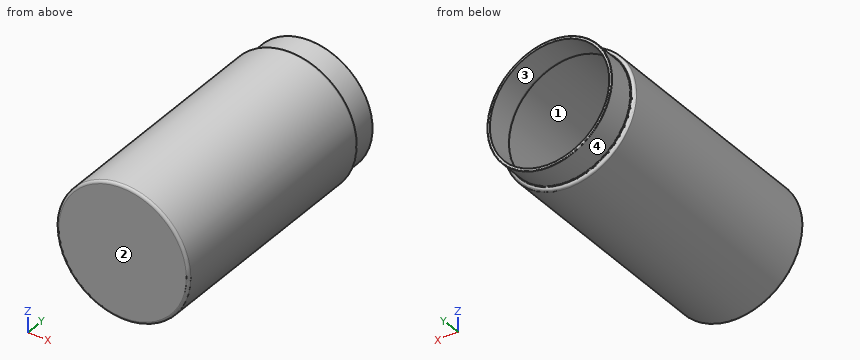
from build123d import *

# Parameters (mm, degrees)
SKETCH1_R           = 25
BOSS_EXTRUDE1_DEPTH = 90
SKETCH2_R           = 23.5
BOSS_EXTRUDE2_DEPTH = 10
FILLET1_R           = 1
FILLET2_R           = 0.2


# Read off the part's stored shape, not the designer's step: Shell1
with BuildPart() as part:
    # Sketch1 → Boss-Extrude1 (new body)
    with BuildSketch(Plane(origin=(0, 0, 0), x_dir=(1, 0, 0), z_dir=(0, 1, 0))):
        with Locations(Location((0, 0, 0), (0, 0, 90))):
            Circle(SKETCH1_R)
    extrude(amount=BOSS_EXTRUDE1_DEPTH)

    # Sketch2 → Boss-Extrude2 (add)
    with BuildSketch(Plane(origin=(0, 90, 0), x_dir=(1, 0, 0), z_dir=(0, 1, 0))):
        with Locations(Location((0, 0, 0), (0, 0, 270))):
            Circle(SKETCH2_R)
    extrude(amount=BOSS_EXTRUDE2_DEPTH)

    # Fillet1
    fillet1_edges = [part.edges().sort_by_distance(p)[0] for p in [
        (0, 0, 25),
        (0, 90, 25),
    ]]
    fillet(fillet1_edges, radius=FILLET1_R)

    # Fillet2
    fillet2_edges = [part.edges().sort_by_distance(p)[0] for p in [
        (0, 90, -23.5),
        (0, 100, -23.5),
    ]]
    fillet(fillet2_edges, radius=FILLET2_R)

    # Shell1 outline → Shell1 (revolve, cut)
    with BuildSketch(Plane.XY):
        with BuildLine():
            Line((24, 1), (24, 89))
            Line((24, 89), (23.7, 89))
            ThreePointArc((23.7, 89), (22.851471863, 89.351471863), (22.5, 90.2))
            Line((22.5, 90.2), (22.5, 100))
            Line((22.5, 100), (0, 100))
            Line((0, 100), (0, 1))
            Line((0, 1), (24, 1))
        make_face()
    revolve(axis=Axis((0, 0, 0), (0, 1, 0)), mode=Mode.SUBTRACT)


solid = part.part
Input: part model. Units: mm. Frame: model coordinates. Face numbers are marked on the shaded views. Round coordinates to 2 decimals unless told otherwise and drop trailing zeros. Loops run counter-clockwise (first coordinate to the right, second up) from the corner with the lowest first, then second, coordinate; pieces in that order, holes last. Notation, with made-up numbers: (-18, -3) -> (-5, -3) arc R28 cw to (-5, 23) -> close; hole circle Ø4 at (24, 52.5). An arc over 180 degrees is marked (long way). Answer as a JSON object with one key per item and string values. Group by question number.
1) Ray query, L1, parallel to X at y = 93, z = 0; L2, parallel to Y at x = 2, z = 0; L3, parallel to Y at x = -8.5, z = 22.5. Return the intervals inside material, ascending.
2) Section query B-B on y = 13.5. Output: boundary loops of the cut face in (x, z).
3) Section query C-C on x = 0. Output: boundary loops of the cut face in (y, z).
4) Draft query along X for the marked faces 1, 2, 3 and 4. Return one class per face: +X half, -X half, draft (parallel to the pull), parting line (faces both ways), or undercut.
5) Pin query (flat end, axial travel): pin 1 (4 mm diameter, centred on y = 12, z = 3.5, fed in from -X); pin 2 (2 mm diameter, centred on x = -7.5, y = 70.5, fed in from +Z); pin 3 (1.5 mm diameter, centred on x = 2.5, y = 34.5, fed in from +Z). Return the tip coordinate at first contact, or that it passes through.
Reply:
{
 "1": {"L1": "x = -23.5 to -22.5, 22.5 to 23.5", "L2": "y = 0 to 1", "L3": "y = 0 to 90"},
 "2": {"outline": "circle Ø50 at (0, 0); hole circle Ø48 at (0, 0)"},
 "3": {"outline": "(0, -24) arc R1 ccw to (1, -25) -> (89, -25) arc R1 ccw to (90, -24) -> (90, -23.7) arc R0.2 cw to (90.2, -23.5) -> (99.8, -23.5) arc R0.2 ccw to (100, -23.3) -> (100, -22.5) -> (90.2, -22.5) arc R1.2 ccw to (89, -23.7) -> (89, -24) -> (1, -24) -> (1, 24) -> (89, 24) -> (89, 23.7) arc R1.2 ccw to (90.2, 22.5) -> (100, 22.5) -> (100, 23.3) arc R0.2 ccw to (99.8, 23.5) -> (90.2, 23.5) arc R0.2 cw to (90, 23.7) -> (90, 24) arc R1 ccw to (89, 25) -> (1, 25) arc R1 ccw to (0, 24) -> close"},
 "4": {"face 1": "undercut", "face 2": "draft", "face 3": "undercut", "face 4": "parting line"},
 "5": {"pin 1": "stops at x = -24.95", "pin 2": "stops at z = 24.14", "pin 3": "stops at z = 24.94"}
}
